Here's the drawing with two shaded views (mm, measured from the low corner). I have some questions. A direction names the side the tool comes from. Coordinates: 2 decimals unless noted, no trailing zeros. Order: outer loops, then holes, each group sorted by start corner. A loop starts at its lowest first (then second) coordinate and runs counter-clockwise, first axis right, second up. Notation, with made-up numbers: (59, 71.5) -> (64, 71.5) arc R8 ccw to (64, 86.5) -> close; hole circle Ø6 at (4.5, 85). An arc over 180 degrees is marked (long way). Answer in a Markdown table with one row per item. Add a question column.
1. Will these pins go through, and if not, where does the flat tip stop? pin 1 (6 mm diameter, centred on x = 28.5, y = 3.5, fed in from -Z) (3 decimals); pin 2 (3 mm diameter, centred on x = 67.5, z = 19, fed in from +Y); pin 3 (10 mm diameter, centred on x = 71.5, y = 13.5, fed in from -Z) (3 decimals).
2. On a 3-axis mill with a long thin cutter (end or side, diameter ignored), from which of +Z, -Z, +X, -X, +Y, -Y can I reach the whole of each face in a straight line? I mean the marked faces 1 and 2. Say none if no direction works.
3. Imagine slicing it at C-C on y = 16.25. Write out the boundary of the cut face in (x, z).
4. If I drill on line 1 along Y through (x, z) = (8, 67); line 2 along X through (y, z) = (8, 73); line 3 along Z through (x, y) = (56, 22.5), over which ranges is the centre line in solid material (lowest first)? Write a range as [from, to].
5. Imagine slicing it at D-D on y = 9.5. Write out the boundary of the cut face in (x, z) (3 decimals), plus the area to 3 significant figures.
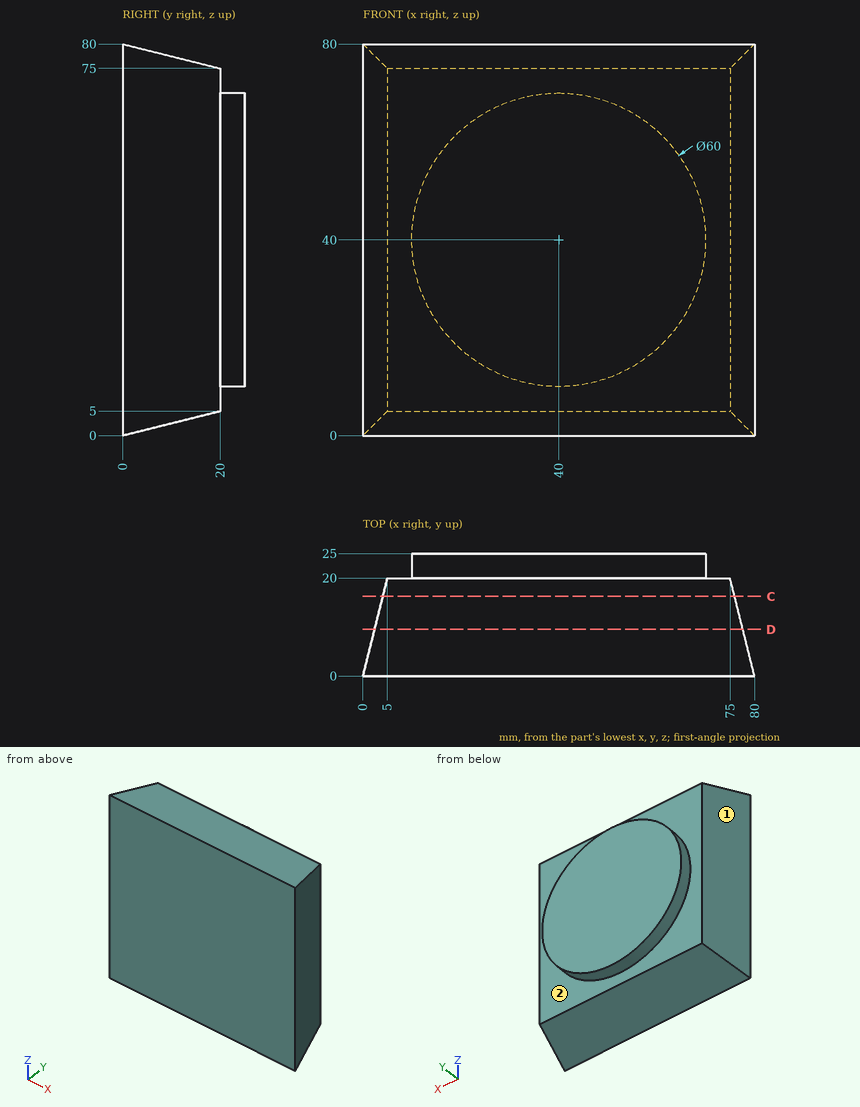
Answers follow:
| question | item | result |
|---|---|---|
| 1 | pin 1 | stops at z = 0.125 |
| 1 | pin 2 | stops at y = 20 |
| 1 | pin 3 | stops at z = 2.125 |
| 2 | face 1 | +Z, -Z, -X, +Y |
| 2 | face 2 | +Y |
| 3 | outline | (4.06, 4.06) -> (75.94, 4.06) -> (75.94, 75.94) -> (4.06, 75.94) -> close |
| 4 | line 1 | y = [0, 20] |
| 4 | line 2 | x = [2, 78] |
| 4 | line 3 | z = [14.62, 65.38] |
| 5 | outline | (2.375, 2.375) -> (77.625, 2.375) -> (77.625, 77.625) -> (2.375, 77.625) -> close |
| 5 | area | 5,660 mm² |
